```python
from build123d import *

# Parameters (mm, degrees)
SKETCH1_R           = 2.7
BOSS_EXTRUDE1_DEPTH = 3.2
CUT_EXTRUDE1_DEPTH  = 2
FILLET1_R           = 0.2
SKETCH3_R           = 1.45
BOSS_EXTRUDE3_DEPTH = 6


with BuildPart() as part:
    # Sketch1 → Boss-Extrude1 (new body)
    with BuildSketch(Plane(origin=(0, 0, 0), x_dir=(1, 0, 0), z_dir=(0, 1, 0))):
        with Locations(Location((0, 0, 0), (0, 0, 270))):
            Circle(SKETCH1_R)
    extrude(amount=BOSS_EXTRUDE1_DEPTH)

    # Sketch2 → Cut-Extrude1 (cut)
    with BuildSketch(Plane(origin=(0, 3.2, 0), x_dir=(1, 0, 0), z_dir=(0, 1, 0))):
        Polygon((1.4, 0), (0.7, 1.212435565), (-0.7, 1.212435565), (-1.4, 0), (-0.7, -1.212435565), (0.7, -1.212435565), align=None)
    extrude(amount=-CUT_EXTRUDE1_DEPTH, mode=Mode.SUBTRACT)

    # Fillet1
    fillet1_edges = [part.edges().sort_by_distance(p)[0] for p in [
        (0, 3.2, -2.7),
    ]]
    fillet(fillet1_edges, radius=FILLET1_R)

    # Sketch3 → Boss-Extrude3 (add)
    with BuildSketch(Plane.XZ):
        with Locations(Location((0, 0, 0), (0, 0, 270))):
            Circle(SKETCH3_R)
    extrude(amount=BOSS_EXTRUDE3_DEPTH)


solid = part.part
```
Source: CAD feature listing. Evaluate the final solid. Frame: model axes, mm. A direction names the side the tool comes from. Round coordinates to 2 decimals unless told otherwise and drop trailing zeros. Loops run counter-clockwise (first coordinate to the right, second up) from the corner with the lowest first, then second, coordinate; pieces in that order, holes last. Notation, with made-up numbers: M 73,72 L 125,72 A16 cw 125,94 Z; hole C 11,83.25 d7. An arc over 180 degrees is marked long. Put each result on its own line as item: value.
(1) First-contact query: pin 1 (1.5 mm diameter, centred on y = -1, z = 2, fed in from -X); pin 2 (1.1 mm diameter, centred on x = 0.5, y = 2.5, fed in from -Z). Flat tips, straight axial feed; report the tip coordinate or a pass-through.
Solutions:
pin 1: x = -0.73
pin 2: z = -2.7
(2) Pull-direction query (X, two-part tool) for faces 1 (the face through (1.055, 2.214, -0.598)), 2 (the face through (0, -6, 0)), 3 (the face through (-1.055, 2.214, 0.598)), 4 (the face through (0.811, 1.479, 2.575)); classes: released by +X, released by -X, zero draft, split by the parting line, or undercut.
Solutions:
face 1: undercut
face 2: zero draft
face 3: undercut
face 4: split by the parting line
(3) Ray query, line 1 (Z direction, x = -0.05, y = 2); line 2 (Y direction, x = 1.95, z = -0.5); line 3 (Z direction, x = -0.9, y = 2). Return the intervals inside material, ascending. Write a range as [from, to].
Solutions:
line 1: [-2.7, -1.21], [1.21, 2.7]
line 2: [0, 3.2]
line 3: [-2.55, -0.87], [0.87, 2.55]
(4) Access query for faces 5 (the face through (0, 2, -1.212)), 6 (the face through (0.06, -2.96, 1.45)), 7 (the face through (-1, 3.2, -1)). Directions: +Z, -Z, +X, -X, +Y, -Y. A direction counts if a zero-diameter tool reaches every point of the face in a straight line with its end or side. Return the directions, or none.
Solutions:
face 5: +Y
face 6: -Y
face 7: +Z, -Z, +X, -X, +Y
(5) Section B-B, the plane y = -5.5. Return loops of the section in (x, z), and give its area (3 significant figures).
Solutions:
outline: C 0,0 d2.9
area: 6.61 mm²
(6) Section A-A, the plane y = 0.5. Return loops of the section in (x, z), and give its area (3 significant figures).
Solutions:
outline: C 0,0 d5.4
area: 22.9 mm²
